Solid Edge part; units mm, degrees
sketch "Sketch1" plane through (0, 0, 0) normal (0, 0, 1) x (1, 0, 0)
  line L0 (-10, -37) -> (10, -37)
  line L1 (10, -37) -> (10, 37)
  line L2 (10, 37) -> (-10, 37)
  line L3 (-10, 37) -> (-10, -37)
  dimension "D1" = 10
  dimension "D2" = 10
extrude "Protrusion1" add sketch "Sketch1" along normal blind 2
sketch "Sketch2" plane through (0, 0, 2) normal (0, 0, 1) x (1, 0, 0)
  line L0 (-10, 37) -> (10, 37)
  line L1 (10, 37) -> (10, -37)
  line L2 (10, -37) -> (-10, -37)
  line L3 (-10, -37) -> (-10, 37)
  line L4 (-8, -35) -> (8, -35)
  line L5 (8, -35) -> (8, 35)
  line L6 (8, 35) -> (-8, 35)
  line L7 (-8, 35) -> (-8, -35)
extrude "Extrusionsausprägung_2" add sketch "Sketch2" along normal blind 10
fillet "Verrundung_3" radius 5 4 edges at (-10, -37, 6) (10, -37, 6) (-10, 37, 6) (10, 37, 6)
fillet "Verrundung_4" radius 2 8 edges at (10, 0, 12) (8.5355, -35.5355, 12) (0, -37, 12) (-8.5355, -35.5355, 12) (-10, 0, 12) (-8.5355, 35.5355, 12) (0, 37, 12) (8.5355, 35.5355, 12)
sketch "Sketch3" plane through (0, 0, 2) normal (0, 0, 1) x (0, -1, 0)
  circle A0 centre (-27, 0) radius 5
  circle A1 centre (27, 0) radius 5
extrude "Cutout1" cut sketch "Sketch3" against normal through all
sketch "Sketch4" plane through (0, 0, 0) normal (0, 0, -1) x (0, -1, 0)
  line L0 (-25.4388, 4.75) -> (-17.4388, 4.75)
  line L1 (-17.4388, 4.75) -> (-17.4388, -4.75)
  line L2 (-17.4388, -4.75) -> (-25.4388, -4.75)
  line L3 (-25.4388, -4.75) -> (-25.4388, 4.75)
  line L4 (25.4388, 4.75) -> (17.4388, 4.75)
  line L5 (17.4388, 4.75) -> (17.4388, -4.75)
  line L6 (17.4388, -4.75) -> (25.4388, -4.75)
  line L7 (25.4388, -4.75) -> (25.4388, 4.75)
  dimension "D1" = 25.4388
  dimension "D2" = 25.4388
extrude "Cutout2" cut sketch "Sketch4" against normal through all
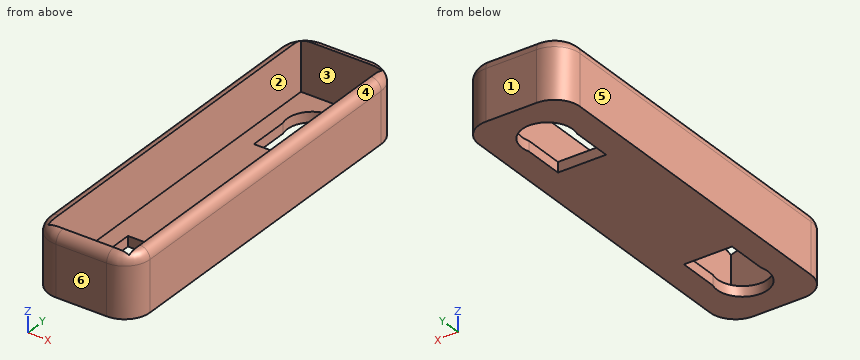
Verification items for the finished model (mm, model axes). Face numbers are marked on the shaded views. A direction names the side the tool comes from. Give positions to 0.01 mm unless a question says otherwise; leave off trailing zeros. Loops run counter-clockwise (first coordinate to the right, second up) from the corner with the lowest first, then second, coordinate; pieces in that order, holes last.
1) Set-up check for the marked faces 1 and 2: record each of +Z, -Z, +X, -X, +Y, -Y from which the full face is reachable in a straight line by a thin tool's end or side.
2) Sectioned sample at A-A, the plane x = 0. Enter the section's corners in (y, z).
3) Depth check by flat-ended pin: pin 1 Ø5 at (x, y) = (0, 10) entering from +Z; pin 2 Ø9 at (x, y) = (0, -27) entering from -Z. Enter the tip coordinate at first touch or a pass-through.
4) Draft check along X on the marked faces 3, 4, 5 and 6. Enter one of: pulls with the +X half, pulls with the -X half, needs draft (parallel to the pull), parting line crosses it, or undercut.
5) Sectioned sample at C-C, the plane z = 5. Enter the section's corners in (x, y), then the cut area to 3 significant figures.
6) Sectioned sample at D-D, the plane y = -14.5. Enter the section's corners in (x, z).
7) Sectioned sample at B-B, the plane y = 27. Enter the section's corners in (x, z).
8) Thickness scan on line 1 along X through (y, z) = (-21, 7.25); line 2 along Y through (x, z) = (-4, 4.5); line 3 along X through (y, z) = (27, 0.8). Record the ranges inside material, lowest first.
Answers:
1. face 1: +Z, -Z, +X, -X, +Y
1. face 2: +Z
2. outline: (-37, 0) - (-32, 0) - (-32, 2) - (-35, 2) - (-35, 12) arc R2 ccw to (-37, 10) - close; (-17.44, 0) - (17.44, 0) - (17.44, 2) - (-17.44, 2) - close; (32, 0) - (37, 0) - (37, 10) arc R2 ccw to (35, 12) - (35, 2) - (32, 2) - close
3. pin 1: stops at z = 2
3. pin 2: passes through
4. face 3: undercut
4. face 4: pulls with the +X half
4. face 5: pulls with the -X half
4. face 6: needs draft
5. outline: (-10, -32) arc R5 ccw to (-5, -37) - (5, -37) arc R5 ccw to (10, -32) - (10, 32) arc R5 ccw to (5, 37) - (-5, 37) arc R5 ccw to (-10, 32) - close; hole (-8, -35) - (8, -35) - (8, 35) - (-8, 35) - close
5. area: 339 mm2
6. outline: (-10, 0) - (10, 0) - (10, 10) arc R2 ccw to (8, 12) - (8, 2) - (-8, 2) - (-8, 12) arc R2 ccw to (-10, 10) - close
7. outline: (-10, 0) - (-5, 0) - (-5, 2) - (-8, 2) - (-8, 12) arc R2 ccw to (-10, 10) - close; (5, 0) - (10, 0) - (10, 10) arc R2 ccw to (8, 12) - (8, 2) - (5, 2) - close
8. line 1: x = -10 to -8, 8 to 10
8. line 2: y = -37 to -35, 35 to 37
8. line 3: x = -10 to -5, 5 to 10
